from build123d import *

# Parameters (mm, degrees)
SKETCH_2_R      = 1.5
SKETCH_2_R_2    = 1
EXTRUDE_1_DEPTH = 0.5
SKETCH_1_R      = 1.5
SKETCH_1_R_2    = 1
EXTRUDE_2_DEPTH = 0.5
SKETCH_3_W      = 17
SKETCH_3_H      = 11
EXTRUDE_3_DEPTH = 0.5


with BuildPart() as part:
    # Sketch 2 → Extrude 1 (new body)
    with BuildSketch(Plane.XY.offset(10)):
        with BuildLine():
            Line((15, 5), (-15, 5))
            Line((-15, 5), (-15, -5))
            Line((-15, -5), (15, -5))
            ThreePointArc((15, -5), (20, 0), (15, 5))
        make_face()
        with Locations((15, 0)):
            Circle(SKETCH_2_R, mode=Mode.SUBTRACT)
        with Locations((2, 0)):
            Circle(SKETCH_2_R_2, mode=Mode.SUBTRACT)
        with Locations((-4, 0)):
            Circle(SKETCH_2_R_2, mode=Mode.SUBTRACT)
        with Locations((-10, 0.253438211)):
            Circle(SKETCH_2_R_2, mode=Mode.SUBTRACT)
    extrude(amount=EXTRUDE_1_DEPTH)



with BuildPart() as body_2:
    # Sketch 1 → Extrude 2 (new body)
    with BuildSketch(Plane.XY):
        with BuildLine():
            Line((-15, 5), (15, 5))
            ThreePointArc((15, 5), (20, 0), (15, -5))
            Line((15, -5), (-15, -5))
            Line((-15, -5), (-15, 5))
        make_face()
        with Locations((15, 0)):
            Circle(SKETCH_1_R, mode=Mode.SUBTRACT)
        with Locations((-10, 0.253438211)):
            Circle(SKETCH_1_R_2, mode=Mode.SUBTRACT)
        with Locations((-4, 0)):
            Circle(SKETCH_1_R_2, mode=Mode.SUBTRACT)
        with Locations((2, 0)):
            Circle(SKETCH_1_R_2, mode=Mode.SUBTRACT)
    extrude(amount=-EXTRUDE_2_DEPTH)


with BuildPart() as part_1:
    add(part.part)

    add(body_2.part)  # Extrude 3 merges body 2
    # Sketch 3 → Extrude 3 (add)
    with BuildSketch(Plane(origin=(0, -5, 0), x_dir=(-1, 0, 0), z_dir=(0, -1, 0))):
        with Locations((6.5, -5)):
            Rectangle(SKETCH_3_W, SKETCH_3_H)
    extrude(amount=EXTRUDE_3_DEPTH)


solid = part_1.part
Geometry: final body of the model. Coordinates: model frame, mm. A direction names the side the tool comes from. Round coordinates to 2 decimals unless told otherwise and drop trailing zeros. Order: outer loops, then holes, each group sorted by start corner. A loop starts at its lowest first (then second) coordinate and runs counter-clockwise, first axis right, second up.
Q1. Pin query (flat end, axial travel): pin 1 (2.5 mm diameter, centred on x = 15, y = 0, fed in from +Z); pin 2 (6 mm diameter, centred on y = -2.5, z = 1.5, fed in from +X); pin 3 (6 mm diameter, centred on y = -4, z = 4.5, fed in from +X); pin 4 (0.6 mm diameter, centred on x = 10.5, z = -0.5, fed in from -Y). Return the tip coordinate at first contact, or that it passes through.
Result sheet:
pin 1: passes through
pin 2: stops at x = 20
pin 3: stops at x = 2
pin 4: stops at y = -5
Q2. Section A-A, the plane y = -3. Output: boundary loops of the cut face in (x, z).
Result sheet:
outline: (-15, -0.5) - (19, -0.5) - (19, 0) - (-15, 0) - close; (-15, 10) - (19, 10) - (19, 10.5) - (-15, 10.5) - close
Q3. Mould query, pull axis Y, two halves, no side actions, for faces 1 (the face through (3, 1, -0.5)), 2 (the face through (-6, -5, 5)), 3 (the face through (13.5, 0.07, -0.25)). Classes: released by +Y, released by -Y, zero draft, split by the parting line, or undercut.
Result sheet:
face 1: zero draft
face 2: released by +Y
face 3: undercut
Q4. Access query for faces 4 (the face through (3, -1, 0)), 5 (the face through (-6, -5.5, 5)). Directions: +Z, -Z, +X, -X, +Y, -Y. A direction counts if a zero-diameter tool reaches every point of the face in a straight line with its end or side. Return the directions, or none.
Result sheet:
face 4: +X, -X, +Y
face 5: +Z, -Z, +X, -X, -Y
Q5. Material intervals for probe 1 along Z at (x, y) = (9, -2); probe 2 along Y at (x, z) = (15, 10.45); probe 3 along Y at (x, z) = (-10, -0.2), sorted ascending.
Result sheet:
probe 1: z = -0.5 to 0, 10 to 10.5
probe 2: y = -5 to -1.5, 1.5 to 5
probe 3: y = -5.5 to -0.75, 1.25 to 5
Q6. Section C-C, the plane z = 3. Output: boundary loops of the cut face in (x, y).
Result sheet:
outline: (-15, -5.5) - (2, -5.5) - (2, -5) - (-15, -5) - close
Q7. Section B-B, the plane x = -4. Output: boundary loops of the cut face in (y, z).
Result sheet:
outline: (-5.5, -0.5) - (-1, -0.5) - (-1, 0) - (-5, 0) - (-5, 10) - (-1, 10) - (-1, 10.5) - (-5.5, 10.5) - close; (1, -0.5) - (5, -0.5) - (5, 0) - (1, 0) - close; (1, 10) - (5, 10) - (5, 10.5) - (1, 10.5) - close
